from build123d import *

# Parameters (mm, degrees)
BOSS_EXTRUDE1_DEPTH = 12.7
SKETCH7_R           = 1.6
CUT_EXTRUDE2_DEPTH  = 12.7
CIRPATTERN1_COUNT   = 3
CUT_EXTRUDE3_DEPTH  = 11.684
CIRPATTERN2_COUNT   = 3
CUT_EXTRUDE5_DEPTH  = 0.7
FILLET2_R           = 2.54


with BuildPart() as part:
    # Sketch1 → Boss-Extrude1 (new body)
    with BuildSketch(Plane(origin=(0, 0, 0), x_dir=(1, 0, 0), z_dir=(0, 1, 0))):
        Polygon((11.43, -19.797340731), (22.86, 0), (11.43, 19.797340731), (-11.43, 19.797340731), (-22.86, 0), (-11.43, -19.797340731), align=None)
    extrude(amount=BOSS_EXTRUDE1_DEPTH)

    # Sketch5 → Cut-Revolve1 (revolve, cut)
    with BuildSketch(Plane(origin=(0, 12.7, 0), x_dir=(1, 0, 0), z_dir=(0, 1, 0))):
        Polygon((0, -19.797340731), (0, -4.672340739), (-3.81, -4.672340739), (-3.81, -10.797340731), (-11.300000006, -10.797340731), (-11.300000006, -17.797340731), (-6.5, -17.797340731), (-6.5, -19.797340731), align=None)
    cut_revolve1 = revolve(axis=Axis((0, 12.7, 19.797340731), (0, 0, -1)), mode=Mode.SUBTRACT)

    # Sketch7 → Cut-Extrude2 (cut)
    with BuildSketch(Plane(origin=(0, 12.7, 0), x_dir=(1, 0, 0), z_dir=(0, 1, 0))):
        with Locations(Location((0, 10.16, 0), (0, 0, 270))):
            Circle(SKETCH7_R)
        with Locations(Location((8.798818102, -5.08, 0), (0, 0, 270))):
            Circle(SKETCH7_R)
        with Locations(Location((-8.798818102, -5.08, 0), (0, 0, 270))):
            Circle(SKETCH7_R)
    extrude(amount=-CUT_EXTRUDE2_DEPTH, mode=Mode.SUBTRACT)

    # CirPattern1: Cut-Revolve1 ×3 about axis
    cirpattern1_axis = Axis((0, 0, 0), (0, 1, 0))
    for i in range(1, CIRPATTERN1_COUNT):
        add(cut_revolve1.rotate(cirpattern1_axis, i * 360 / CIRPATTERN1_COUNT), mode=Mode.SUBTRACT)

    # Sketch8 → Cut-Extrude3 (cut)
    with BuildSketch(Plane.XY.offset(19.797340731)):
        with BuildLine():
            Line((-13.856406592, 12.7), (-18.662949192, 12.7))
            Line((-18.662949192, 12.7), (-18.662949192, 0))
            Line((-18.662949192, 0), (18.662949192, 0))
            Line((18.662949192, 0), (18.662949192, 12.7))
            Line((18.662949192, 12.7), (13.856406592, 12.7))
            ThreePointArc((13.856406592, 12.7), (0, 0.69999987), (-13.856406592, 12.7))
        make_face()
    cut_extrude3 = extrude(amount=-CUT_EXTRUDE3_DEPTH, mode=Mode.SUBTRACT)

    # CirPattern2: Cut-Extrude3 ×3 about axis
    cirpattern2_axis = Axis((0, 0, 0), (0, 1, 0))
    for i in range(1, CIRPATTERN2_COUNT):
        add(cut_extrude3.rotate(cirpattern2_axis, i * 360 / CIRPATTERN2_COUNT), mode=Mode.SUBTRACT)

    # Sketch10 → Cut-Extrude5 (cut)
    with BuildSketch(Plane.XZ):
        Polygon((14.052718364, 8.113340731), (-14.052718364, 8.113340731), (0, -16.226681461), align=None)
    extrude(amount=-CUT_EXTRUDE5_DEPTH, mode=Mode.SUBTRACT)

    # Fillet2
    # the kernel refuses this fillet: 2.54 mm, written as the material it takes off along each edge
    with BuildSketch(Plane(origin=(14.052718364, -10.298522628, 8.113340731), x_dir=(-0.4999999999999996, 0, -0.8660254037844387), z_dir=(0, 1, 0))) as fillet2_piece_1_section:
        with BuildLine():
            CenterArc((FILLET2_R * 1.73205080757, FILLET2_R), FILLET2_R, 150, 120)
            Line((FILLET2_R * 0.866025403784, FILLET2_R * 1.5), (0, 0))
            Line((0, 0), (FILLET2_R * 1.73205080757, 0))
        make_face()
    fillet2_piece_1 = extrude(amount=33.997045256, mode=Mode.PRIVATE)
    fillet2_piece_1 = fillet2_piece_1 - Plane(origin=(6.277314066, 14.7, -3.624208966), x_dir=(-0.49487165940112743, -0.14285714153061227, -0.8571428573086736), z_dir=(0.8660254037844388, 0, -0.49999999999999983)) * Cylinder(14.00000013, 86, mode=Mode.PRIVATE)
    fillet2_piece_1 = fillet2_piece_1 - Plane(origin=(0, 14.7, 7.248417919), x_dir=(0.9897433188022552, -0.14285714153061224, 0), z_dir=(0, 0, 1)) * Cylinder(14.00000013, 86, mode=Mode.PRIVATE)
    add(fillet2_piece_1, mode=Mode.SUBTRACT)
    with BuildSketch(Plane(origin=(0, -10.298522628, -16.226681461), x_dir=(-0.5000000000000003, 0, 0.8660254037844386), z_dir=(0, 1, 0))) as fillet2_piece_2_section:
        with BuildLine():
            CenterArc((FILLET2_R * 1.73205080757, FILLET2_R), FILLET2_R, 150, 120)
            Line((FILLET2_R * 0.866025403784, FILLET2_R * 1.5), (0, 0))
            Line((0, 0), (FILLET2_R * 1.73205080757, 0))
        make_face()
    fillet2_piece_2 = extrude(amount=33.997045256, mode=Mode.PRIVATE)
    fillet2_piece_2 = fillet2_piece_2 - Plane(origin=(6.277314055, 14.7, -3.62420896), x_dir=(-0.49487165940112743, -0.14285714153061227, -0.8571428573086736), z_dir=(0.8660254037844388, 0, -0.49999999999999983)) * Cylinder(14.00000013, 86, mode=Mode.PRIVATE)
    fillet2_piece_2 = fillet2_piece_2 - Plane(origin=(-6.277314066, 14.7, -3.624208966), x_dir=(-0.4948716594011281, -0.14285714153061227, 0.8571428573086732), z_dir=(-0.8660254037844384, 0, -0.5000000000000004)) * Cylinder(14.00000013, 86, mode=Mode.PRIVATE)
    add(fillet2_piece_2, mode=Mode.SUBTRACT)
    with BuildSketch(Plane(origin=(-14.052718364, 23.698522628, 8.113340731), x_dir=(1, 0, 0), z_dir=(0, -1, 0))) as fillet2_piece_3_section:
        with BuildLine():
            CenterArc((FILLET2_R * 1.73205080757, -FILLET2_R), FILLET2_R, 90, 120)
            Line((FILLET2_R * 0.866025403784, -FILLET2_R * 1.5), (0, 0))
            Line((0, 0), (FILLET2_R * 1.73205080757, 0))
        make_face()
    fillet2_piece_3 = extrude(amount=33.997045256, mode=Mode.PRIVATE)
    fillet2_piece_3 = fillet2_piece_3 - Plane(origin=(0, 14.7, 7.248417932), x_dir=(0.9897433188022552, -0.14285714153061224, 0), z_dir=(0, 0, 1)) * Cylinder(14.00000013, 86, mode=Mode.PRIVATE)
    fillet2_piece_3 = fillet2_piece_3 - Plane(origin=(-6.277314055, 14.7, -3.62420896), x_dir=(-0.4948716594011281, -0.14285714153061227, 0.8571428573086732), z_dir=(-0.8660254037844384, 0, -0.5000000000000004)) * Cylinder(14.00000013, 86, mode=Mode.PRIVATE)
    add(fillet2_piece_3, mode=Mode.SUBTRACT)


solid = part.part
Check sheet for the modelled part. Datum: model origin and axes. Units: mm. A direction names the side the tool comes from. Give positions to 0.01 mm unless a question says otherwise; leave off trailing zeros. Loops run counter-clockwise (first coordinate to the right, second up) from the corner with the lowest first, then second, coordinate; pieces in that order, holes last. Notation, with made-up numbers: M 1.25,53 L 57.25,53 A22 ccw 57.25,86 Z; hole C 22.25,-35.5 d7. An arc over 180 degrees is marked long. Use a Markdown table: item, result. Add a question column.
Q1. Go/stop test with flat-tipped pins: pin 1 (1.1 mm diameter, centred on x = -0.5, y = 11.5, fed in from +Z); pin 2 (5 mm diameter, centred on y = 2.5, z = -6, fed in from +X); pin 3 (2 mm diameter, centred on y = 4.5, z = -3, fed in from -X); pin 4 (3 mm diameter, centred on x = -8.8, z = 5.08, fed in from -Y). Record where each tip stops, or that it passes through.
Q2. Tool access check on faces 4 (the flat face through (0, 7, 10.797)), 5 (the cylindrical face through (-11.83, 3.29, 6.88)), 6 (the cylindrical face through (0.037, 3.201, -13.686)). Record the directions out of +Z, -Z, +X, -X, +Y, -Y that give a thin tool (end or side, any length) a straight path to the whole face; none if there is none.
Q3. Mould release check, pull along Z, two halves, no side actions. Record for faces 1 (the flat face through (-9.27, 7.13, -5.54)), 2 (the flat face through (0, 11, 4.672)), 3 (the flat face through (-10, 10, -19.797)): pulls with the +Z half, pulls with the -Z half, needs draft (parallel to the pull), parting line crosses it, or undercut.
Q4. Scan lines: line 1 along X through (y, z) = (11, -2); line 2 along X through (y, z) = (11, 3); line 3 along Z through (x, y) = (3, 12.25). Record each from-to range of solid material in increasing order. Write a range as [from, to].
Q5. Sectioned sample at A-A, the plane y = 5.25. Record the cut outline in (x, z), then the cut area to 3 significant figures.
Q6. Sectioned sample at B-B, the plane z = 5.5. Give the number of separate pieces and of enclosed holes in the cut face, then the cut area to 3 significant figures.
Verdict:
| question | item | result |
|---|---|---|
| 1 | pin 1 | z = 4.67 |
| 1 | pin 2 | x = 20.83 |
| 1 | pin 3 | x = -21.71 |
| 1 | pin 4 | through |
| 2 | face 4 | +Y |
| 2 | face 5 | -X, -Y |
| 2 | face 6 | -Z, -Y |
| 3 | face 1 | undercut |
| 3 | face 2 | pulls with the +Z half |
| 3 | face 3 | pulls with the -Z half |
| 4 | line 1 | [-21.71, -19.4], [-11.31, -10.28], [-4.24, 4.24], [10.28, 11.31], [19.4, 21.71] |
| 4 | line 2 | [-21.13, -17.15], [-14.2, 14.2], [17.15, 21.13] |
| 4 | line 3 | [-17.65, -6.1], [-4.15, 4.67] |
| 5 | outline | M -22.31,-0.95 L -11.98,-18.84 L -1.78,-12.96 A2.54 ccw 1.78,-12.96 L 11.98,-18.84 L 22.31,-0.95 L 12.11,4.93 A2.54 ccw 10.33,8.02 L 10.33,19.8 L -10.33,19.8 L -10.33,8.02 A2.54 ccw -12.11,4.93 Z; hole M -19.66,-1.54 L -11.16,-16.26 L -5.1,-12.76 L -13.6,1.96 Z; hole C -8.8,5.08 d3.2; hole M -8.5,10.8 L 8.5,10.8 L 8.5,17.8 L -8.5,17.8 Z; hole C 0,-10.16 d3.2; hole M 5.1,-12.76 L 11.16,-16.26 L 19.66,-1.54 L 13.6,1.96 Z; hole C 8.8,5.08 d3.2 |
| 5 | area | 672 mm^2 |
| 6 | separate pieces | 3 |
| 6 | enclosed holes | 0 |
| 6 | area | 247 mm^2 |
